from build123d import *

# Parameters (mm, degrees)
F0_W     = 10
F0_H     = 10
F1_DEPTH = 1
F2_R     = 2.5
F3_DEPTH = 2
F4_R     = 2
F5_R     = 0.5


with BuildPart() as f1:
    # F0 (on Top) → F1 (new body)
    with BuildSketch(Plane.XY):
        with Locations((-5, 5)):
            Rectangle(F0_W, F0_H)
    extrude(amount=F1_DEPTH)

    # F2 (on Top) → F3 (join)
    with BuildSketch(Plane.XY):
        with Locations((-9, 9)):
            Circle(F2_R)
    extrude(amount=F3_DEPTH)

    # F4
    f4_edges = [f1.edges().sort_by_distance(p)[0] for p in [
        (0, 10, 0.5),
        (0, 0, 0.5),
        (-10, 0, 0.5),
    ]]
    fillet(f4_edges, radius=F4_R)

    # F5
    f5_edges = [f1.edges().sort_by_distance(p)[0] for p in [
        (-10, 4.354356, 1),
        (-11.5, 9, 2),
    ]]
    fillet(f5_edges, radius=F5_R)


solid = f1.part
Can you work these out from the model? Positions are in its coordinate system, mm. A direction names the side the tool comes from. Coordinates: 2 decimals unless noted, no trailing zeros. Loops run counter-clockwise (first coordinate to the right, second up) from the corner with the lowest first, then second, coordinate; pieces in that order, holes last. Notation, with made-up numbers: M 6.5,-36.5 L 36.5,-36.5 A12 ccw 36.5,-24.5 Z; hole C 38,51.25 d8. An arc over 180 degrees is marked long. Return JSON: item names as keys, results as strings. Group by question number.
Item 1: I'm going to push flat-ended pins straight in: pin 1 Ø2.5 at (x, y) = (-6, 3) entering from +Z; pin 2 Ø0.6 at (y, z) = (4.5, 0.5) entering from -X. Where does each tip first touch, or does it pass through?
Item 2: Imagine slicing it at A-A (z = 0.3). Please give me the cut outline in (x, y), and give its area (3 significant figures).
Item 3: If I drill on L1, parallel to Z at x = -2.5, y = 8.5; L2, parallel to X at y = 7.5, z = 1.5; L3, parallel to Y at x = -4.25, z = 0.35, over which ranges is the centre line in solid material (lowest first)? Write a range as from..to.
Item 4: Imagine slicing it at B-B (y = 4.75). Please give me the cut outline in (x, z).
Item 5: On a 3-axis mill with a long thin cutter (end or side, diameter ignored), from which of +Z, -Z, +X, -X, +Y, -Y can I reach the whole of each face in a straight line? I mean faces 1 (the flat face through (-5, 5, 1)), 2 (the cylindrical face through (-10.84, 10.69, 0.91)), 3 (the cylindrical face through (-0.57, 0.6, 0.25)). Say none if no direction works.
Verdict:
{
 "1": {"pin 1": "stops at z = 1", "pin 2": "stops at x = -10"},
 "2": {"outline": "M -10,2 A2 ccw -8,0 L -2,0 A2 ccw 0,2 L 0,8 A2 ccw -2,10 L -6.71,10 A2.5 ccw long -10,6.71 Z", "area": "106 mm^2"},
 "3": {"L1": "z = 0..1", "L2": "x = -11..-7", "L3": "y = 0..10"},
 "4": {"outline": "M -10,0 L 0,0 L 0,0.5 A0.5 ccw -0.5,1 L -9.5,1 A0.5 ccw -10,0.5 Z"},
 "5": {"face 1": "+Z, +X, -Y", "face 2": "+Z", "face 3": "+Z, -Z, +X, -Y"}
}
